Input: part model. Units: mm. Frame: model coordinates. Face numbers are marked on the shaded views. Coordinates: 2 decimals unless noted, no trailing zeros. Write each loop counter-clockwise with the first axis right and the second up, starting at its lowest first coordinate (ties: lowest second). Pieces come first, ordered by that corner, then holes. Notation, with made-up numbers: M 11,70.25 L 56,70.25 A30 cw 56,95.25 Z; hole C 25.5,44.5 d6. An arc over 180 degrees is marked long. Answer as a JSON object with one key per item and string values. Group by question number.
from build123d import *

# Parameters (mm, degrees)
SKETCH3_R          = 2.0828
CUT_EXTRUDE1_DEPTH = 12.169052528
CHAMFER1_SIZE      = 0.1984375


with BuildPart() as part:
    # Sketch1 → Revolve1 (revolve)
    with BuildSketch(Plane.XY, mode=Mode.PRIVATE) as revolve1_sk:
        with BuildLine():
            Line((0, 7.9375), (-4.7625, 7.9375))
            Line((-4.7625, 7.9375), (-4.7625, 7.46125))
            ThreePointArc((-4.7625, 7.46125), (-3.81, 5.318125), (-4.7625, 3.175))
            Line((-4.7625, 3.175), (-5.55625, 3.175))
            Line((-5.55625, 3.175), (-5.55625, 0))
            Line((-5.55625, 0), (0, 0))
            Line((0, 0), (0, 7.9375))
        make_face()
    revolve(revolve1_sk.sketch.rotate(Axis((0, 0, 0), (0, 1, 0)), 270), axis=Axis((0, 0, 0), (0, 1, 0)))

    # Sketch3 → Cut-Extrude1 (cut, through all)
    with BuildSketch(Plane(origin=(0, 0, 0), x_dir=(1, 0, 0), z_dir=(0, 1, 0))):
        with Locations(Location((0, 0, 0), (0, 0, 270))):
            Circle(SKETCH3_R)
    extrude(amount=CUT_EXTRUDE1_DEPTH, mode=Mode.SUBTRACT)

    # Chamfer1
    chamfer1_edges = [part.edges().sort_by_distance(p)[0] for p in [
        (0, 0, 5.55625),
        (0, 3.175, 5.55625),
    ]]
    chamfer(chamfer1_edges, length=CHAMFER1_SIZE)


solid = part.part
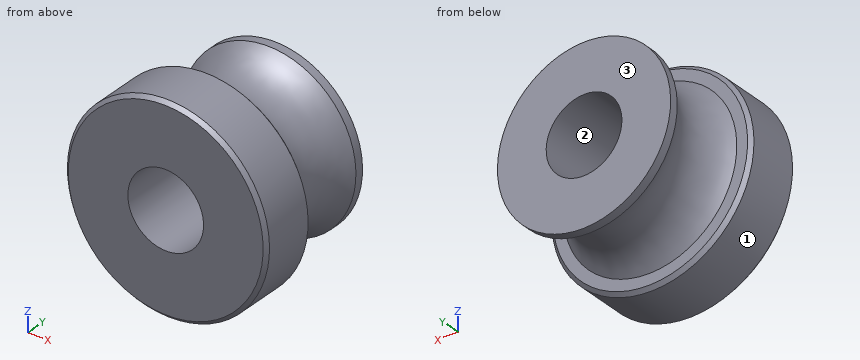
Q1. Line query: line 1 (X direction, y = 6, z = 0.5); line 2 (X direction, y = 4.5, z = 0); line 3 (Y direction, x = -2.75, z = 3). Output: solid intervals per line, ascending. Write a range as from..to.
Q2. Section D-D, the plane y = 5. Return the cut outline in (x, z).
Q3. Section C-C, the plane y = 6.5. Return the cut outline in (x, z).
Q4. Draft query along X for the marked faces 1, 2 and 3. Return one class per face: released by +X, released by -X, zero draft, split by the parting line, or undercut.
Q5. Pin query (flat end, axial travel): pin 1 Ø1.5 at (x, z) = (-4, 2.5) entering from -Y; pin 2 Ø1.5 at (x, y) = (2, 1.5) entering from -Z; pin 3 Ø1.5 at (y, z) = (3, -1) entering from -X. Return the tip coordinate at first contact, or that it passes through.
Filled in:
{
 "1": {"line 1": "-3.86..-2.02, 2.02..3.86", "line 2": "-3.93..-2.08, 2.08..3.93", "line 3": "0..4.12, 6.51..7.94"},
 "2": {"outline": "C 0,0 d7.66; hole C 0,0 d4.17"},
 "3": {"outline": "C 0,0 d8.13; hole C 0,0 d4.17"},
 "4": {"face 1": "split by the parting line", "face 2": "undercut", "face 3": "zero draft"},
 "5": {"pin 1": "y = 0", "pin 2": "z = -5.41", "pin 3": "x = -5.55"}
}
